```python
from build123d import *

# Parameters (mm, degrees)
SKETCH_1_R      = 7.5
EXTRUDE_1_DEPTH = 18
SKETCH_2_R      = 23
SKETCH_2_R_2    = 15
EXTRUDE_2_DEPTH = 20
EXTRUDE_3_DEPTH = 9


with BuildPart() as part:
    # Sketch 1 → Extrude 1 (new body)
    with BuildSketch(Plane(origin=(0, 0, 0), x_dir=(1, 0, 0), z_dir=(0, 1, 0))):
        with BuildLine():
            Line((-57.92, -20.52495067), (-14.4, -37.318092127))
            ThreePointArc((-14.4, -37.318092127), (0, -40), (14.4, -37.318092127))
            Line((14.4, -37.318092127), (57.92, -20.52495067))
            ThreePointArc((57.92, -20.52495067), (72, 0), (57.92, 20.52495067))
            Line((57.92, 20.52495067), (14.4, 37.318092127))
            ThreePointArc((14.4, 37.318092127), (0, 40), (-14.4, 37.318092127))
            Line((-14.4, 37.318092127), (-57.92, 20.52495067))
            ThreePointArc((-57.92, 20.52495067), (-72, 0), (-57.92, -20.52495067))
        make_face()
        with Locations((50, 0)):
            Circle(SKETCH_1_R, mode=Mode.SUBTRACT)
        with Locations((-50, 0)):
            Circle(SKETCH_1_R, mode=Mode.SUBTRACT)
    extrude(amount=EXTRUDE_1_DEPTH)



with BuildPart() as body_2:
    # Sketch 2 → Extrude 2 (new body, symmetric)
    with BuildSketch(Plane(origin=(0, 0, 0), x_dir=(0, 0, -1), z_dir=(1, 0, 0))):
        with Locations((0, 76)):
            Circle(SKETCH_2_R)
        with Locations((0, 76)):
            Circle(SKETCH_2_R_2, mode=Mode.SUBTRACT)
    extrude(amount=EXTRUDE_2_DEPTH, both=True)


with BuildPart() as part_1:
    add(part.part)

    add(body_2.part)  # Extrude 3 merges body 2
    # Sketch 2_3 → Extrude 3 (add, symmetric)
    with BuildSketch(Plane(origin=(0, 0, 0), x_dir=(0, 0, -1), z_dir=(1, 0, 0))):
        with BuildLine():
            ThreePointArc((23, 76), (-1.989918559, 53.08624378), (-22.655671663, 79.964913806))
            Line((-22.655671663, 79.964913806), (-33.5, 18))
            Line((-33.5, 18), (33.5, 18))
            Line((33.5, 18), (22.655671663, 79.964913806))
            ThreePointArc((22.655671663, 79.964913806), (22.91375622, 77.989918559), (23, 76))
        make_face()
    extrude(amount=EXTRUDE_3_DEPTH, both=True)


solid = part_1.part
```
Here's how the part is built. I have some questions about the finished solid (model axes, mm). A direction names the side the tool comes from. Give positions to 0.01 mm unless a question says otherwise; leave off trailing zeros. Order: outer loops, then holes, each group sorted by start corner. A loop starts at its lowest first (then second) coordinate and runs counter-clockwise, first axis right, second up. Notation, with made-up numbers: (-4, 2.5) - (32, 2.5) arc R18 cw to (32, 30.5) - close; hole circle Ø4 at (7, -38.5). An arc over 180 degrees is marked (long way). Answer as a JSON object with one key per item and string values. Group by question number.
Item 1: For P1, Ø14, axis at y = 73.5, z = -4, coming from the -X side; P2, Ø3, axis at x = 23.5, z = -15, coming from the +Y side; P3, Ø5, axis at y = 34, z = 6.5, coming from the -X side; P4, Ø8, axis at y = 35, z = -11, coming from the +X side, each with a flat end and sliding along its axis, tell me the tip position at first contact or that it passes through.
Item 2: If we section it at C-C on y = 76: Please give me the cut outline in (x, z).
Item 3: Which directions (+Z, -Z, +X, -X, +Y, -Y) give clear straight access to the entire face, cutting with the end or side of a thin tool? Please do faces 4 (the cylindrical face through (-0.28, 61.357, 3.252)), 5 (the flat face through (-20, 61, -5)).
Item 4: If we section it at B-B on z = 0: Please give me the cut outline in (x, y), and give its area (3 significant figures).
Item 5: Please list where these lines run through material, in increasing order: probe 1 along X at (y, z) = (8, 0); probe 2 along Y at (x, z) = (19.5, 0.5); probe 3 along Y at (x, z) = (30.5, 24).
Item 6: If we section it at D-D on x = 17: Please give me the cut outline in (y, z), and give its area (3 significant figures).
Item 7: If we section it at A-A on x = -50: Please give me the cut outline in (y, z), and give its area (3 significant figures).
Item 8: If we mould it in two halves opening along Y, with no side actions, what happens to faces 1 (the flat face through (0.126, 48.549, -28.154)), 2 (the flat face through (36.465, 8.874, -28.804)), 3 (the cylindrical face through (0.28, 98.804, 2.994))? For each: pulls with the +Y half, pulls with the -Y half, needs draft (parallel to the pull), parting line crosses it, or undercut.
Result set:
{
 "1": {"P1": "through", "P2": "y = 18", "P3": "x = -9", "P4": "x = 9"},
 "2": {"outline": "(-20, -23) - (-9, -23) - (-9, -23.35) - (9, -23.35) - (9, -23) - (20, -23) - (20, -15) - (-20, -15) - close; (-20, 15) - (20, 15) - (20, 23) - (9, 23) - (9, 23.35) - (-9, 23.35) - (-9, 23) - (-20, 23) - close"},
 "3": {"face 4": "+X, -X", "face 5": "+Z, -Z, -X, +Y"},
 "4": {"outline": "(-72, 0) - (-57.5, 0) - (-57.5, 18) - (-72, 18) - close; (-42.5, 0) - (42.5, 0) - (42.5, 18) - (9, 18) - (9, 53) - (20, 53) - (20, 61) - (-20, 61) - (-20, 53) - (-9, 53) - (-9, 18) - (-42.5, 18) - close; (-20, 91) - (20, 91) - (20, 99) - (-20, 99) - close; (57.5, 0) - (72, 0) - (72, 18) - (57.5, 18) - close", "area": "3,320 mm²"},
 "5": {"probe 1": "-72 to -57.5, -42.5 to 42.5, 57.5 to 72", "probe 2": "0 to 18, 53.01 to 61.01, 90.99 to 98.99", "probe 3": "0 to 18"},
 "6": {"outline": "(0, -36.31) - (18, -36.31) - (18, 36.31) - (0, 36.31) - close; circle Ø46 at (76, 0); hole circle Ø30 at (76, 0)", "area": "2,260 mm²"},
 "7": {"outline": "(0, -23.58) - (18, -23.58) - (18, -7.5) - (0, -7.5) - close; (0, 7.5) - (18, 7.5) - (18, 23.58) - (0, 23.58) - close", "area": "579 mm²"},
 "8": {"face 1": "pulls with the +Y half", "face 2": "needs draft", "face 3": "undercut"}
}
